from build123d import *

# Parameters (mm, degrees)
SKETCH1_R           = 2.286
BOSS_EXTRUDE1_DEPTH = 19.05
SKETCH2_W           = 72.350889222
SKETCH2_H           = 23.78555394
CUT_EXTRUDE1_DEPTH  = 2.54


with BuildPart() as part:
    # Sketch1 → Boss-Extrude1 (new body)
    with BuildSketch(Plane.XY):
        with BuildLine():
            Line((-44.45, -36.5125), (44.45, -36.5125))
            ThreePointArc((44.45, -36.5125), (48.940128061, -34.652628061), (50.8, -30.1625))
            Line((50.8, -30.1625), (50.8, 30.1625))
            ThreePointArc((50.8, 30.1625), (48.940128061, 34.652628061), (44.45, 36.5125))
            Line((44.45, 36.5125), (-44.45, 36.5125))
            ThreePointArc((-44.45, 36.5125), (-48.940128061, 34.652628061), (-50.8, 30.1625))
            Line((-50.8, 30.1625), (-50.8, -30.1625))
            ThreePointArc((-50.8, -30.1625), (-48.940128061, -34.652628061), (-44.45, -36.5125))
        make_face()
        with Locations(Location((-45.632054244, 22.9235, 0), (0, 0, 180))):
            Circle(SKETCH1_R, mode=Mode.SUBTRACT)
        with Locations(Location((45.72, 22.9235, 0), (0, 0, 180))):
            Circle(SKETCH1_R, mode=Mode.SUBTRACT)
        with Locations(Location((45.72, -23.0505, 0), (0, 0, 180))):
            Circle(SKETCH1_R, mode=Mode.SUBTRACT)
        with Locations(Location((-45.632054244, -23.0505, 0), (0, 0, 180))):
            Circle(SKETCH1_R, mode=Mode.SUBTRACT)
    extrude(amount=BOSS_EXTRUDE1_DEPTH)

    # Sketch2 → Cut-Extrude1 (cut)
    with BuildSketch(Plane.XY.offset(19.05)):
        Rectangle(SKETCH2_W, SKETCH2_H)
    extrude(amount=-CUT_EXTRUDE1_DEPTH, mode=Mode.SUBTRACT)


solid = part.part
Can you work these out from the model? Positions are in its coordinate system, mm. A direction names the side the tool comes from. Give positions to 0.01 mm unless a question says otherwise; leave off trailing zeros. Order: outer loops, then holes, each group sorted by start corner. A loop starts at its lowest first (then second) coordinate and runs counter-clockwise, first axis right, second up. Notation, with made-up numbers: M 75,83.25 L 120,83.25 A11 ccw 120,96.25 Z; hole C 49,44.25 d10. An arc over 180 degrees is marked long. Use a Markdown table: item, result. Add a question column.
Item 1: For faces 5 (the flat face through (-1, 17, 19.05)), 6 (the flat face through (36.175, 0, 18)), which set-ups out of +Z, -Z, +X, -X, +Y, -Y let a thin tool reach every point of the face, with its end or its side?
Item 2: Suppose I cut it at A-A (x = -0.5). List the corners of the cut face in (y, z) for me, then the cut area to 3 significant figures.
Item 3: We'd pull the mould along Y, two halves only. Please class faces 1 (the flat face through (-1, 11.893, 18)), 2 (the flat face through (1, 36.512, 9)), 3 (the flat face through (-1, -36.512, 9)), 4 (the flat face through (50.8, 0, 9)): +Y half, -Y half, draft (parallel to the pull), parting line (faces both ways), or undercut.
Item 4: If I drill on L1, parallel to Y at x = 23.5, z = 17.5; L2, parallel to X at y = -23, z = 17.5; L3, parallel to Y at x = 45.72, z = 9.25, over which ranges is the centre line in solid material (lowest first)? Write a range as [from, to].
Item 5: Suppose I cut it at B-B (x = 45.72). List the corners of the cut face in (y, z) for me.
Item 6: Will this pin go through, and if not, where does the flat tip stop? pin 1 (2.5 mm diameter, centred on x = -45.63, y = -23.05, fed in from +Z).
Answer sheet:
| question | item | result |
|---|---|---|
| 1 | face 5 | +Z, +X, -X, +Y, -Y |
| 1 | face 6 | +Z |
| 2 | outline | M -36.51,0 L 36.51,0 L 36.51,19.05 L 11.89,19.05 L 11.89,16.51 L -11.89,16.51 L -11.89,19.05 L -36.51,19.05 Z |
| 2 | area | 1,330 mm² |
| 3 | face 1 | undercut |
| 3 | face 2 | +Y half |
| 3 | face 3 | -Y half |
| 3 | face 4 | draft |
| 4 | L1 | y = [-36.51, -11.89], [11.89, 36.51] |
| 4 | L2 | x = [-50.8, -47.92], [-43.35, 43.43], [48.01, 50.8] |
| 4 | L3 | y = [-36.38, -25.34], [-20.76, 20.64], [25.21, 36.38] |
| 5 | outline | M -36.38,0 L -25.34,0 L -25.34,19.05 L -36.38,19.05 Z; M -20.76,0 L 20.64,0 L 20.64,19.05 L -20.76,19.05 Z; M 25.21,0 L 36.38,0 L 36.38,19.05 L 25.21,19.05 Z |
| 6 | pin 1 | passes through |
